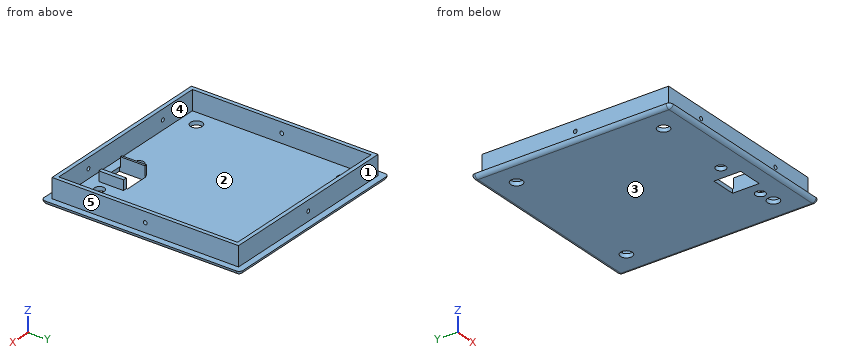
Autodesk Inventor part; units mm, degrees
ref_plane "YZ Plane" through (0, 0, 0) normal (1, 0, 0) x (0, 1, 0)
ref_plane "XZ Plane" through (0, 0, 0) normal (0, 1, 0) x (-1, 0, 0)
ref_plane "XY Plane" through (0, 0, 0) normal (0, 0, 1) x (1, 0, 0)
sketch "Skizze1" plane through (0, 0, 0) normal (0, 0, 1) x (1, 0, 0)
  line L0 (-50.8, 50.8) -> (50.8, 50.8)
  line L1 (50.8, 50.8) -> (50.8, -50.8)
  line L2 (50.8, -50.8) -> (-50.8, -50.8)
  line L3 (-50.8, -50.8) -> (-50.8, 50.8)
  line L4 (50.8, -50.8) -> (-50.8, 50.8) construction
  point P0 (0, 0)
  point P1 (0, 0)
  dimension "d0" = 101.6
  dimension "d1" = 101.6
extrude "Extrusion1" add sketch "Skizze1" against normal blind 2.0066
fillet "Rundung1" radius 2.0066 4 edges at (50.8, -50.8, -1.0033) (50.8, 50.8, -1.0033) (-50.8, 50.8, -1.0033) (-50.8, -50.8, -1.0033)
fillet "Rundung2" radius 2.0066 8 edges at (-50.2123, -50.2123, -2.0066) (-50.8, 0, -2.0066) (-50.2123, 50.2123, -2.0066) (0, 50.8, -2.0066) (50.2123, 50.2123, -2.0066) (50.8, 0, -2.0066) (50.2123, -50.2123, -2.0066) (0, -50.8, -2.0066)
sketch "Skizze2" plane through (0, 0, 0) normal (0, 0, 1) x (1, 0, 0)
  line L0 (-47.5996, 47.5996) -> (47.5996, 47.5996)
  line L1 (47.5996, 47.5996) -> (47.5996, -47.5996)
  line L2 (47.5996, -47.5996) -> (-47.5996, -47.5996)
  line L3 (-47.5996, -47.5996) -> (-47.5996, 47.5996)
  line L4 (47.5996, -47.5996) -> (-47.5996, 47.5996) construction
  line L5 (-45.593, 45.593) -> (45.593, 45.593)
  line L6 (45.593, 45.593) -> (45.593, -45.593)
  line L7 (45.593, -45.593) -> (-45.593, -45.593)
  line L8 (-45.593, -45.593) -> (-45.593, 45.593)
  line L9 (-45.593, -45.593) -> (45.593, 45.593) construction
  point P0 (0, 0)
  point P1 (0, 0)
  dimension "d6" = 95.1992
  dimension "d7" = 2.0066
extrude "Extrusion2" add sketch "Skizze2" along normal blind 9.9822
sketch "Skizze3" plane through (47.5996, -47.5996, 0) normal (1, 0, 0) x (0, 0, -1)
  line L0 (0, 95.1992) -> (0, 0)
  line L1 (0, 95.1992) -> (-9.9822, 95.1992)
  line L2 (-9.9822, 0) -> (-9.9822, 95.1992)
  line L3 (0, 0) -> (-9.9822, 0)
  line L4 (0, 47.5996) -> (-4.7752, 47.5996) construction
  line L5 (0, 95.1992) -> (0, 0) construction
  dimension "d10" = 4.7752
hole "Bohrung1" at (47.5996, 0, 4.7752) direction (-1, 0, 0) diameter 1.941 depth 7.675 tip angle 118
pattern_circular "Runde Anordnung1" count 3 over 180 about axis through (0, 0, -10) along (0, 0, 1) of "Bohrung1"
sketch "Skizze4" plane through (-47.5996, -47.5996, 0) normal (0, -1, 0) x (1, 0, 0)
  line L0 (95.1992, 0) -> (0, 0)
  line L1 (95.1992, 0) -> (95.1992, 9.9822)
  line L2 (0, 9.9822) -> (95.1992, 9.9822)
  line L3 (0, 0) -> (0, 9.9822)
  line L4 (47.5996, 0) -> (47.5996, 4.7752) construction
  line L5 (22.1996, 4.7752) -> (72.9996, 4.7752) construction
  dimension "d21" = 4.7752
  dimension "d22" = 50.8
hole "Bohrung2" at (-25.4, -47.5996, 4.7752) at (25.4, -47.5996, 4.7752) direction (0, 1, 0) diameter 1.941 depth 7.675 tip angle 118
sketch "Skizze5" plane through (0, 0, -2.0066) normal (0, 0, -1) x (-1, 0, 0)
  line L0 (37.5031, -37.5031) -> (-37.5031, -37.5031) construction
  line L1 (-37.5031, -37.5031) -> (-37.5031, 37.5031) construction
  line L2 (-37.5031, 37.5031) -> (37.5031, 37.5031) construction
  line L3 (37.5031, 37.5031) -> (37.5031, -37.5031) construction
  line L4 (-37.5031, 37.5031) -> (37.5031, -37.5031) construction
  point P0 (0, 0)
  point P1 (0, 0)
  dimension "d30" = 75.0062
hole "Bohrung3" at (-37.5031, 37.5031, -2.0066) direction (0, 0, 1) diameter 6 end through all
sketch "Skizze6" plane through (0, 0, 0) normal (0, 0, 1) x (1, 0, 0)
  circle A0 centre (-37.5031, 37.5031) radius 3
  line L0 (-48.7934, 48.7934) -> (-48.7934, -48.7934)
  line L1 (48.7934, 48.7934) -> (-48.7934, 48.7934)
  line L2 (48.7934, -48.7934) -> (48.7934, 48.7934)
  line L3 (-48.7934, -48.7934) -> (48.7934, -48.7934)
  circle A1 centre (-37.5031, 37.5031) radius 3.45
  circle A2 centre (-37.5031, 37.5031) radius 1.4986
  point P0 (0, 0)
  dimension "d38" = 2.9972
  dimension "d39" = 6.9
extrude "Extrusion3" add sketch "Skizze6" along normal blind 5 contours A0 | A1
pattern_circular "Runde Anordnung2" count 4 over 360 about axis through (0, 0, -10) along (0, 0, 1) of "Bohrung3", "Extrusion3"
sketch "Skizze7" plane through (0, 0, 0) normal (0, 0, 1) x (1, 0, 0)
  circle A0 centre (37.5031, 37.5031) radius 3
  circle A1 centre (37.5031, -37.5031) radius 3
  circle A2 centre (-37.5031, -37.5031) radius 3
  circle A3 centre (-37.5031, 37.5031) radius 3
  line L0 (-48.7934, 48.7934) -> (-48.7934, -48.7934)
  line L1 (48.7934, 48.7934) -> (-48.7934, 48.7934)
  line L2 (48.7934, -48.7934) -> (48.7934, 48.7934)
  line L3 (-48.7934, -48.7934) -> (48.7934, -48.7934)
  line L4 (7.9248, -28.2956) -> (24.638, -28.2956)
  line L5 (24.638, -28.2956) -> (24.638, -44.2214)
  line L6 (24.638, -44.2214) -> (7.9248, -44.2214)
  line L7 (7.9248, -44.2214) -> (7.9248, -28.2956)
  line L8 (9.9314, -30.3022) -> (22.6314, -30.3022)
  line L9 (22.6314, -30.3022) -> (22.6314, -43.0022)
  line L10 (22.6314, -43.0022) -> (9.9314, -43.0022)
  line L11 (9.9314, -43.0022) -> (9.9314, -30.3022)
  line L12 (16.2814, -28.2956) -> (16.2814, -30.3022) construction
  circle A4 centre (2.7814, -36.6522) radius 1.4986
  circle A5 centre (2.7814, -36.6522) radius 3.4163
  circle A6 centre (29.7814, -36.6522) radius 1.4986
  circle A7 centre (29.7814, -36.6522) radius 3.4163
  line L13 (9.9314, -43.0022) -> (22.6314, -30.3022) construction
  line L14 (29.7814, -36.6522) -> (2.7814, -36.6522) construction
  line L15 (50.8, -48.7934) -> (48.7934, -48.7934)
  arc A8 (48.7934, -50.8) -> (50.8, -48.7934) centre (48.7934, -48.7934) ccw
  line L16 (48.7934, -48.7934) -> (48.7934, -50.8)
  line L17 (50.8, 48.7934) -> (50.8, -48.7934)
  line L18 (48.7934, -50.8) -> (-48.7934, -50.8)
  point P0 (0, 0)
  point P1 (16.2814, -36.6522)
  dimension "d46" = 12.7
  dimension "d49" = 1.2192
  dimension "d51" = 6.8326
  dimension "d52" = 27
  dimension "d53" = 2.9972
  dimension "d58" = 2.0066
  dimension "d59" = 2.0066
  dimension "d61" = 14.1478
  dimension "d70" = 28.1686
  dimension "d71" = 21.0186
  dimension "d72" = 27
extrude "Extrusion4" add sketch "Skizze7" along normal blind 5.0038 contours L4 L5 L6 L7 | A4 | A5 | A6 | A7
sketch "Skizze8" plane through (0, 0, -2.0066) normal (0, 0, -1) x (-1, 0, 0)
  circle A0 centre (-29.7814, -36.6522) radius 2.5019
  circle A1 centre (-2.7814, -36.6522) radius 2.5019
  circle A2 centre (-2.7814, -36.6522) radius 3.4163
  circle A3 centre (-29.7814, -36.6522) radius 3.4163
  point P0 (0, 0)
  dimension "d64" = 5.0038
extrude "Extrusion5" cut sketch "Skizze8" against normal blind 2.0066 contours A0 | A1
sketch "Skizze10" plane through (2.7814, -36.6522, 5.0038) normal (0, 0, 1) x (1, 0, 0)
  circle A0 centre (0, 0) radius 3.4163
  circle A1 centre (27, 0) radius 3.4163
  circle A2 centre (0, 0) radius 1.5875
  circle A3 centre (27, 0) radius 3.4163
  circle A4 centre (27, 0) radius 1.5875
  point P0 (-2.7814, 36.6522)
  dimension "d67" = 3.175
extrude "Extrusion6" cut sketch "Skizze10" against normal blind 3.4798 contours A2 | A4
sketch "Skizze12" plane through (0, 0, 9.9822) normal (0, 0, 1) x (1, 0, 0)
  line L0 (45.593, -45.593) -> (45.593, 45.593) construction
  line L1 (45.593, 45.593) -> (-45.593, 45.593) construction
  line L2 (-45.593, 45.593) -> (-45.593, -45.593) construction
  line L3 (-45.593, -45.593) -> (45.593, -45.593) construction
  circle A0 centre (-37.5031, 37.5031) radius 3.45 construction
  circle A1 centre (-37.5031, -37.5031) radius 3.45 construction
  circle A2 centre (37.5031, -37.5031) radius 3.45 construction
  circle A3 centre (37.5031, 37.5031) radius 3.45 construction
  circle A4 centre (29.7814, -36.6522) radius 3.4163 construction
  circle A5 centre (2.7814, -36.6522) radius 3.4163 construction
  line L4 (24.638, -28.2956) -> (24.638, -44.2214) construction
  line L5 (24.638, -44.2214) -> (7.9248, -44.2214) construction
  line L6 (7.9248, -44.2214) -> (7.9248, -28.2956) construction
  line L7 (7.9248, -28.2956) -> (24.638, -28.2956) construction
  line L8 (-47.625, 47.625) -> (47.625, 47.625) construction
  line L9 (47.625, 47.625) -> (47.625, -47.625) construction
  line L10 (47.625, -47.625) -> (-47.625, -47.625) construction
  line L11 (-47.625, -47.625) -> (-47.625, 47.625) construction
  line L12 (47.625, -47.625) -> (-47.625, 47.625) construction
  line L13 (45.593, -45.593) -> (-45.593, -45.593) construction
  line L14 (-45.593, 45.593) -> (45.593, 45.593) construction
  line L15 (-45.593, -45.593) -> (45.593, 45.593) construction
  line L16 (9.9314, -27.775) -> (22.6314, -27.775)
  line L17 (22.6314, -27.775) -> (22.6314, -41.375)
  line L18 (22.6314, -41.375) -> (9.9314, -41.375)
  line L19 (9.9314, -41.375) -> (9.9314, -27.775)
  line L20 (22.6314, -30.3022) -> (22.6314, -43.0022)
  line L21 (9.9314, -43.0022) -> (9.9314, -30.3022)
  circle A6 centre (37.5031, 37.5031) radius 1.4986
  circle A7 centre (37.5031, 37.5031) radius 3.45
  circle A8 centre (37.5031, -37.5031) radius 1.4986
  circle A9 centre (37.5031, -37.5031) radius 3.45
  circle A10 centre (29.7814, -36.6522) radius 1.5875
  circle A11 centre (29.7814, -36.6522) radius 3.4163
  line L22 (7.9248, -28.2956) -> (7.9248, -44.2214)
  line L23 (24.638, -28.2956) -> (24.638, -44.2214)
  line L24 (7.9248, -44.2214) -> (24.638, -44.2214)
  line L25 (24.638, -44.2214) -> (24.638, -40.875)
  line L26 (24.638, -40.875) -> (7.9248, -40.875)
  line L27 (7.9248, -40.875) -> (7.9248, -44.2214)
  line L28 (7.9248, -28.2956) -> (8.9248, -28.2956)
  line L29 (8.9248, -28.2956) -> (8.9248, -40.875)
  line L30 (8.9248, -40.875) -> (7.9248, -40.875)
  line L31 (7.9248, -40.875) -> (7.9248, -28.2956)
  circle A12 centre (2.7814, -36.6522) radius 1.5875
  circle A13 centre (2.7814, -36.6522) radius 3.4163
  circle A14 centre (-37.5031, -37.5031) radius 3
  circle A15 centre (-37.5031, -37.5031) radius 3.45
  circle A16 centre (-37.5031, 37.5031) radius 1.4986
  circle A17 centre (-37.5031, 37.5031) radius 3.45
  point P0 (0, 0)
  point P1 (0, 0)
  point P2 (16.2814, -41.375)
  dimension "d76" = 95.25
  dimension "d77" = 12.7
  dimension "d78" = 13.6
  dimension "d79" = 6.25
  dimension "d80" = 63.9064
  dimension "d84" = 1
  dimension "d87" = 2.8464
  dimension "d88" = 3.3464
extrude "Extrusion7" cut sketch "Skizze12" against normal through all contours L16 L17 L26 L19 | L26 L17 L18 L19
extrude "Extrusion8" cut sketch "Skizze12" against normal up to surface (9.9822 mm away) contours L26 L17 L18 L19 | L19 L18 L17 L26 L23 L24 L22 | L26 L22 L28 L29 | A7 | A9 | A10 | A11 | A12 | A13 | A14 | A15 | A17
equation "\"d59\" = d58"
properties part number "Nanolab CubeDeckel 2"
Work out the finished part from the listing and answer in its coordinate system (mm). Face numbers are marked on the shaded views. A direction names the side the tool comes from. Give positions to 0.01 mm unless a question says otherwise; leave off trailing zeros. Order: outer loops, then holes, each group sorted by start corner. A loop starts at its lowest first (then second) coordinate and runs counter-clockwise, first axis right, second up. Notation, with made-up numbers: (68.25, 41) - (72.25, 41) arc R35 cw to (72.25, 75) - close; hole circle Ø4 at (12, -16.5). An arc over 180 degrees is marked (long way). One line per item, written item: value. Start each with the question number.
1. Consider line 1 (Y direction, x = -31, z = 8.5); line 2 (Z direction, x = -5.5, y = 29). Determine where each line is inside the solid, lowest interval first.
2. Section B-B, the plane z = 7 is taken. Write down the section's boundary in (x, y).
3. For a pull along Y with two mould halves and no side action, classify the marked faces 1, 2 and 3 as released by +Y, released by -Y, zero draft, split by the parting line, or undercut.
4. Which of the six approach directions +Z, -Z, +X, -X, +Y, -Y give full straight-line access (tool end or side, diameter ignored) to the marked faces 4 and 5?
5. Each of these flat-tipped pins is pushed along its axis until it touches: pin 1 Ø4.5 at (x, y) = (2.78, -36.65) entering from -Z; pin 2 Ø5 at (y, z) = (-29.5, 5.5) entering from -X; pin 3 Ø1 at (x, z) = (16, -1.5) entering from -Y; pin 4 Ø1 at (x, z) = (17.5, -1) entering from +Y. Where does it stop, or does it pass through?
Filled sheet:
1. line 1: -47.6 to -45.59, 45.59 to 47.6
1. line 2: -2.01 to 0
2. outline: (-47.6, -47.6) - (47.6, -47.6) - (47.6, 47.6) - (-47.6, 47.6) - close; hole (-45.59, -45.59) - (45.59, -45.59) - (45.59, 45.59) - (-45.59, 45.59) - close
3. face 1: released by +Y
3. face 2: undercut
3. face 3: zero draft
4. face 4: +Z
4. face 5: +Z, +X, +Y, -Y
5. pin 1: through
5. pin 2: x = -47.6
5. pin 3: y = -50.53
5. pin 4: y = 50.74
